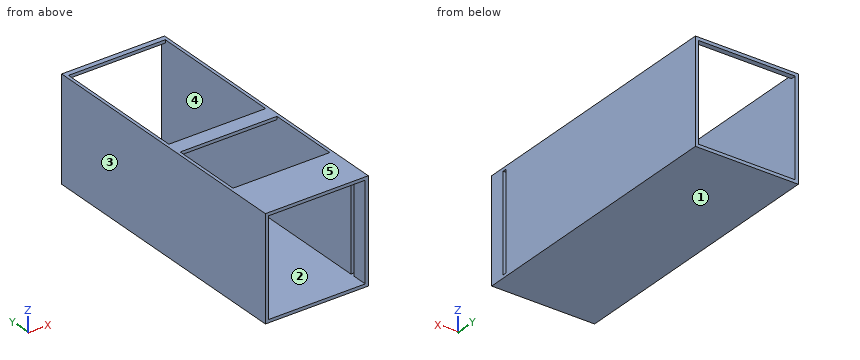
Autodesk Inventor part; units mm, degrees
ref_plane "YZ Plane" through (0, 0, 0) normal (1, 0, 0) x (0, 1, 0)
ref_plane "XZ Plane" through (0, 0, 0) normal (0, 1, 0) x (-1, 0, 0)
ref_plane "XY Plane" through (0, 0, 0) normal (0, 0, 1) x (1, 0, 0)
sketch "Sketch1" plane through (0, 0, 0) normal (0, 1, 0) x (-1, 0, 0)
  line L0 (50, 50) -> (-50, 50)
  line L1 (-50, 50) -> (-50, -50)
  line L2 (-50, -50) -> (50, -50)
  line L3 (50, -50) -> (50, 50)
  line L4 (50, 50) -> (-50, -50) construction
  line L5 (-50, 50) -> (50, -50) construction
  line L6 (-47, 47) -> (47, 47)
  line L7 (47, 47) -> (47, -47)
  line L8 (47, -47) -> (-47, -47)
  line L9 (-47, -47) -> (-47, 47)
  line L10 (-47, 47) -> (47, -47) construction
  line L11 (47, 47) -> (-47, -47) construction
  point P0 (0, 0)
  dimension "d0" = 100
  dimension "d1" = 100
  dimension "d2" = 3
  dimension "d3" = 3
extrude "Extrusion1" add sketch "Sketch1" along normal blind 270
sketch "Sketch2" plane through (-50, 0, 50) normal (0, 0, 1) x (1, 0, 0)
  line L0 (3, 265) -> (97, 265)
  line L1 (97, 265) -> (97, 132)
  line L2 (97, 132) -> (3, 132)
  line L3 (3, 132) -> (3, 265)
  line L4 (0, 0) -> (0, 270)
  line L5 (0, 270) -> (100, 270)
  line L6 (3, 117) -> (97, 117)
  line L7 (97, 117) -> (97, 47)
  line L8 (97, 47) -> (3, 47)
  line L9 (3, 47) -> (3, 117)
  line L10 (100, 0) -> (100, 270)
  point P0 (50, 0)
  point P1 (50, 270)
  point P2 (50, 265)
  dimension "d6" = 94
  dimension "d7" = 3
  dimension "d8" = 5
  dimension "d9" = 133
  dimension "d10" = 70
  dimension "d11" = 15
  dimension "d12" = 3
extrude "Extrusion2" cut sketch "Sketch2" against normal blind 10
sketch "Sketch10" plane through (50, 0, 50) normal (1, 0, 0) x (0, 0, -1)
  line L0 (3, 0) -> (3, 47)
  line L1 (97, 0) -> (97, 270)
  line L2 (3, 19) -> (97, 19)
  line L3 (97, 19) -> (97, 15)
  line L4 (97, 15) -> (3, 15)
  line L5 (3, 15) -> (3, 19)
  line L6 (0, 0) -> (100, 0)
  point P0 (50, 0)
  point P1 (3, 15)
  dimension "d46" = 4
  dimension "d49" = 15
extrude "Extrusion10" cut sketch "Sketch10" against normal blind 10 contours L0 L2 L1 L4
equation "\"d1\" = d0"
equation "\"d12\" = d7"
properties part number "FLU-ShaftRS3" material "Steel"
Read the model definition and answer for the solid it produces. Units are mm, in the model's axes. Face numbers are marked on the shaded views. A direction names the side the tool comes from. Coordinates: 2 decimals unless noted, no trailing zeros. Loops run counter-clockwise (first coordinate to the right, second up) from the corner with the lowest first, then second, coordinate; pieces in that order, holes last. Notation, with made-up numbers: (72.5, -31) - (129.5, -31) arc R30 cw to (129.5, 6) - close; hole circle Ø2 at (32, 28). An arc over 180 degrees is marked (long way). Answer in a Markdown table with one row per item.
Q1. Given P1, Ø1, axis at x = -15, y = 52.5, coming from the +Z side, flat-ended and moving along its own axis, determine where the tip first touches the part or whether it passes through.
Here are the results:
| item | result |
|---|---|
| P1 | stops at z = -47 |
Q2. Find section C-C on y = 64. Write down the section's boundary in (x, z), plus the area to 3 significant figures.
Here are the results:
| item | result |
|---|---|
| outline | (-50, -50) - (50, -50) - (50, 50) - (47, 50) - (47, -47) - (-47, -47) - (-47, 50) - (-50, 50) - close |
| area | 882 mm^2 |
Q3. Straight lines are drawn through the part: line 1 along X through (y, z) = (68, -7.5); line 2 along Z through (x, y) = (45.5, 223.5). For each, find the intervals that lie inside material, in ascending order. Write a range as [from, to].
Here are the results:
| item | result |
|---|---|
| line 1 | x = [-50, -47], [47, 50] |
| line 2 | z = [-50, -47] |
Q4. Find section B-B on x = 6. Write down the section's boundary in (y, z), plus the area to 3 significant figures.
Here are the results:
| item | result |
|---|---|
| outline | (0, -50) - (270, -50) - (270, -47) - (0, -47) - close; (0, 47) - (47, 47) - (47, 50) - (0, 50) - close; (117, 47) - (132, 47) - (132, 50) - (117, 50) - close; (265, 47) - (270, 47) - (270, 50) - (265, 50) - close |
| area | 1,010 mm^2 |
Q5. For the marked faces 1 and 2, determine the directions among +Z, -Z, +X, -X, +Y, -Y from which every point of the face is accessible in a straight line to the end or side of a thin tool.
Here are the results:
| item | result |
|---|---|
| face 1 | -Z, +X, -X, +Y, -Y |
| face 2 | +Y, -Y |
Q6. The mould has two halves that part along Z. Classify the marked faces 3, 4 and 5: pulls with the +Z half, pulls with the -Z half, needs draft (parallel to the pull), parting line crosses it, or undercut.
Here are the results:
| item | result |
|---|---|
| face 3 | needs draft |
| face 4 | undercut |
| face 5 | pulls with the +Z half |
Q7. Find section A-A on z = -1.5. Write down the section's boundary in (x, y).
Here are the results:
| item | result |
|---|---|
| outline | (-50, 0) - (-47, 0) - (-47, 270) - (-50, 270) - close; (47, 0) - (50, 0) - (50, 15) - (47, 15) - close; (47, 19) - (50, 19) - (50, 270) - (47, 270) - close |
